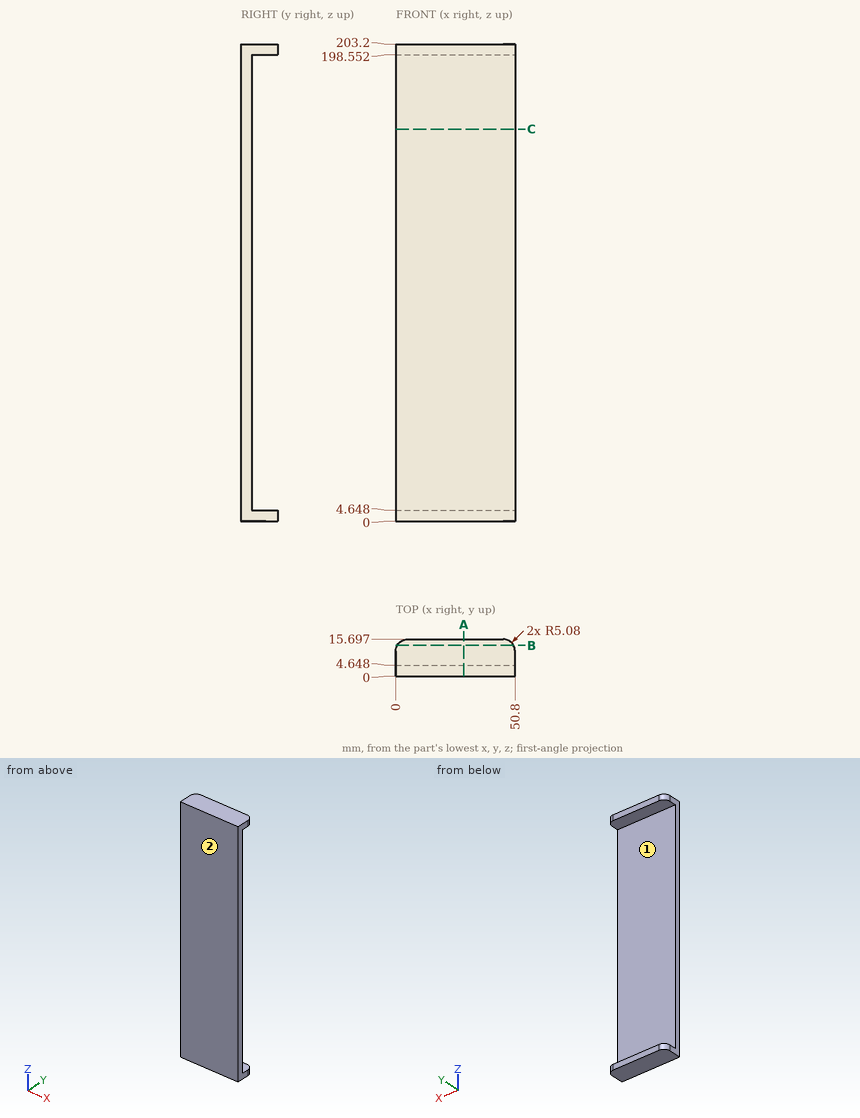
Can you work these out from the drawing? Everything is in mm from the part's minimum corner. A direction names the side the tool comes from. Round coordinates to 2 decimals unless told otherwise and drop trailing zeros. Order: outer loops, then holes, each group sorted by start corner. A loop starts at its lowest first (then second) coordinate and runs counter-clockwise, first axis right, second up. Notation, with made-up numbers: (12.5, -37.5) -> (67.5, -37.5) arc R12 cw to (67.5, -26.5) -> close; hole circle Ø6 at (85, 70). An arc over 180 degrees is marked (long way). Return JSON: item names as keys, results as strings. Group by question number.
1. Will this pin go through, and if not, where does the flat tip stop? pin 1 (5 mm diameter, centred on x = 30, z = 70.5, fed in from +Y).
2. If we section it at A-A, the plane x = 29: Write out the boundary of the cut face in (y, z).
3. If we section it at C-C, the plane z = 167: Write out the boundary of the cut face in (x, y), then the cut area to 3 significant figures.
4. If we section it at B-B, the plane y = 13: Write out the boundary of the cut face in (x, z).
5. I need wall thicknesses on line 1 (Z direction, x = 12, y = 9); line 2 (Y direction, x = 28.5, z = 64.5). Which ranges of each line are inside material? Lowest first, please. Write a range as [from, to].
6. Which directions (+Z, -Z, +X, -X, +Y, -Y) give clear straight access to the entire face, cutting with the end or side of a thin tool? Please do the marked faces 1 and 2.
Output values:
{
 "1": {"pin 1": "y = 4.65"},
 "2": {"outline": "(0, 0) -> (15.7, 0) -> (15.7, 4.65) -> (4.65, 4.65) -> (4.65, 198.55) -> (15.7, 198.55) -> (15.7, 203.2) -> (0, 203.2) -> close"},
 "3": {"outline": "(0, 0) -> (50.8, 0) -> (50.8, 4.65) -> (0, 4.65) -> close", "area": "236 mm²"},
 "4": {"outline": "(0.59, 0) -> (50.21, 0) -> (50.21, 4.65) -> (0.59, 4.65) -> close; (0.59, 198.55) -> (50.21, 198.55) -> (50.21, 203.2) -> (0.59, 203.2) -> close"},
 "5": {"line 1": "[0, 4.65], [198.55, 203.2]", "line 2": "[0, 4.65]"},
 "6": {"face 1": "+X, -X, +Y", "face 2": "+Z, -Z, +X, -X, -Y"}
}
